The figure shows three views and two pictorial views of one solid part (mm, origin at its lowest corner). Answer the questions. Round coordinates to 2 decimals unless told otherwise and drop trailing zeros. Loops run counter-clockwise (first coordinate to the right, second up) from the corner with the lowest first, then second, coordinate; pieces in that order, holes last. Notation, with made-up numbers: (26, 39.5) -> (39, 39.5) arc R19 cw to (39, 59.5) -> close; hole circle Ø3 at (12.5, 89). An arc over 180 degrees is marked (long way). Write item = value, one per line. Start each with the question number.
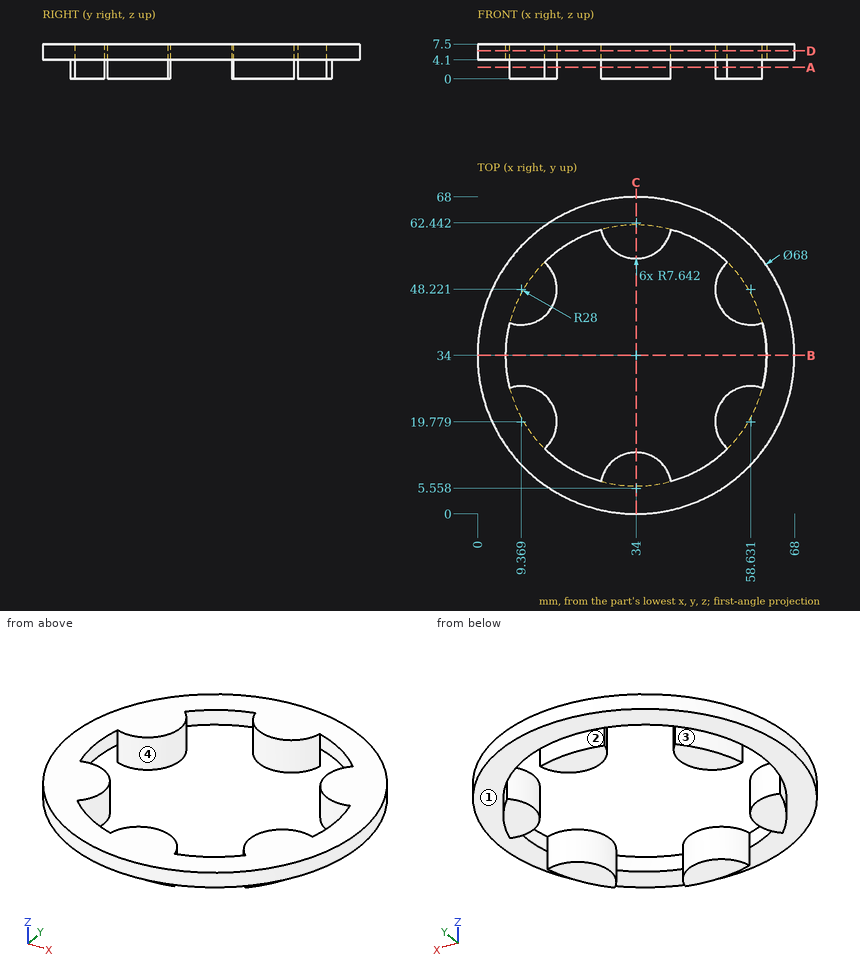
Item 1: Find the intervals of material crossed by line 1 along Y through (x, z) = (53, 6.75) (1 decimal); line 2 along Y through (x, z) = (33.5, 2.5) (1 decimal); line 3 along Z through (x, y) = (42, 65.5), in increasing order. Write a range as [from, to].
Item 2: The mould has two halves that part along X. Classify the marked faces 1, 2, 3 and 4: pulls with the +X half, pulls with the -X half, needs draft (parallel to the pull), parting line crosses it, or undercut.
Item 3: Section B-B (y = 34) is taken. Determine the outline of the cut face in (x, z), then the cut area to 3 significant figures.
Item 4: Flat-ended cylindrical pins translate along their axes: pin 1 (1.5 mm diameter, centred on x = 43, z = 6.5, fed in from +Y); pin 2 (4 mm diameter, centred on x = 37, z = 3.5, fed in from -Y); pin 3 (1.5 mm diameter, centred on x = 60.5, z = 4, fed in from -Y) (1 decimal); pin 4 (3 mm diameter, centred on x = 45.5, z = 2, fed in from +Y). Find the tip coordinate at first contact, or state that the pin passes through.
Item 5: Section D-D (z = 6) is taken. Determine the outline of the cut face in (x, y).
Item 6: Section A-A (z = 2.5) is taken. Determine the outline of the cut face in (x, y).
Item 7: Section C-C (x = 34) is taken. Determine the outline of the cut face in (y, z).
Worked answers:
q1.line_1 = [5.8, 13.4], [14.6, 24.9], [43.1, 53.4], [54.6, 62.2]
q1.line_2 = [6, 13.2], [54.8, 62]
q1.line_3 = [4.1, 7.5]
q2.face_1 = needs draft
q2.face_2 = parting line crosses it
q2.face_3 = pulls with the -X half
q2.face_4 = undercut
q3.outline = (0, 4.1) -> (6, 4.1) -> (6, 7.5) -> (0, 7.5) -> close; (62, 4.1) -> (68, 4.1) -> (68, 7.5) -> (62, 7.5) -> close
q3.area = 40.8 mm2
q4.pin_1 = 66.98
q4.pin_2 = 0.02
q4.pin_3 = 11.8
q4.pin_4 = through
q5.outline = circle Ø68 at (34, 34); hole (6.89, 27.01) arc R7.64 cw to (14.39, 14.02) arc R28 ccw to (26.5, 7.02) arc R7.64 cw to (41.5, 7.02) arc R28 ccw to (53.61, 14.02) arc R7.64 cw to (61.11, 27.01) arc R28 ccw to (61.11, 40.99) arc R7.64 cw to (53.61, 53.98) arc R28 ccw to (41.5, 60.98) arc R7.64 cw to (26.5, 60.98) arc R28 ccw to (14.39, 53.98) arc R7.64 cw to (6.89, 40.99) arc R28 ccw to start
q6.outline = (6.89, 27.01) arc R28 ccw to (14.39, 14.02) arc R7.64 ccw to start; (6.89, 40.99) arc R7.64 ccw to (14.39, 53.98) arc R28 ccw to start; (26.5, 7.02) arc R28 ccw to (41.5, 7.02) arc R7.64 ccw to start; (26.5, 60.98) arc R7.64 ccw to (41.5, 60.98) arc R28 ccw to start; (53.61, 14.02) arc R28 ccw to (61.11, 27.01) arc R7.64 ccw to start; (53.61, 53.98) arc R7.64 ccw to (61.11, 40.99) arc R28 ccw to start
q7.outline = (0, 4.1) -> (6, 4.1) -> (6, 0) -> (13.2, 0) -> (13.2, 7.5) -> (0, 7.5) -> close; (54.8, 0) -> (62, 0) -> (62, 4.1) -> (68, 4.1) -> (68, 7.5) -> (54.8, 7.5) -> close
